Check sheet for the drawn part. Datum: minimum x, y, z corner. Units: mm. A direction names the side the tool comes from. Give positions to 0.01 mm unless a question says otherwise; leave off trailing zeros. Order: outer loops, then holes, each group sorted by start corner. A loop starts at its lowest first (then second) coordinate and runs counter-clockwise, first axis right, second up.
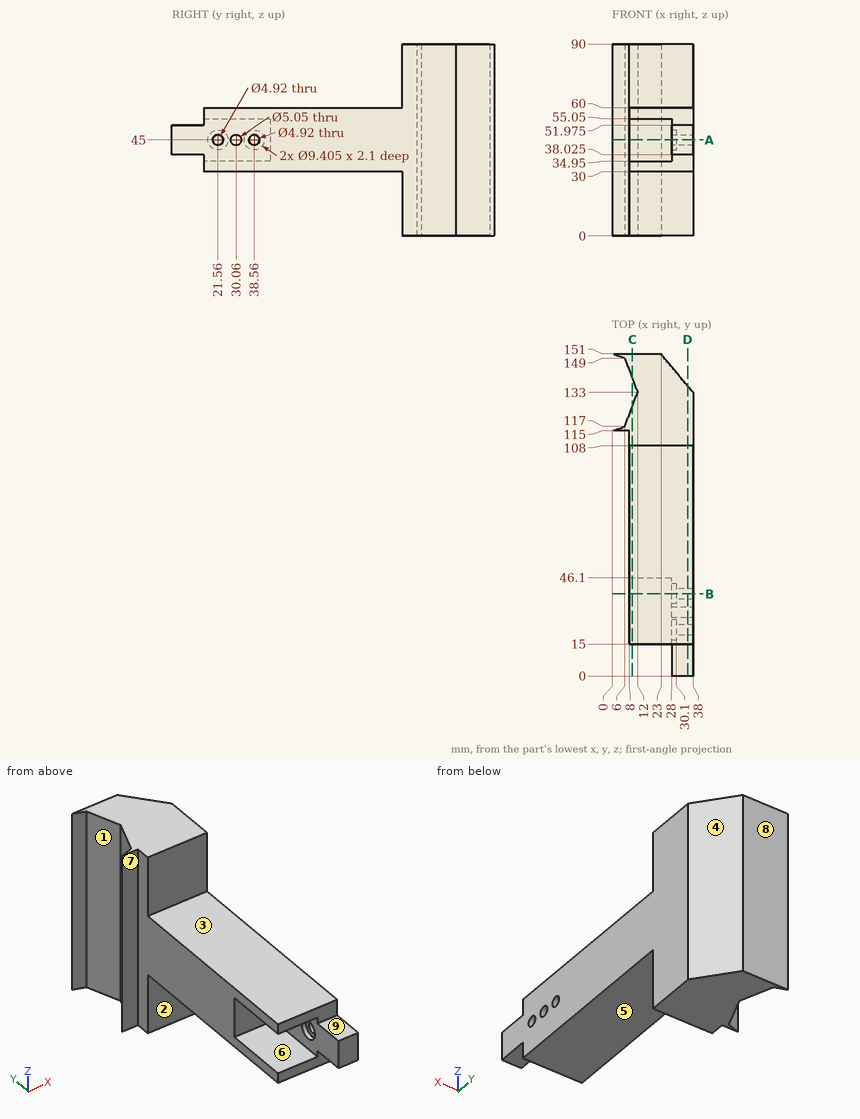
(1) Section check C-C, the plane x = 9.5. Enter the section's corners in (y, z).
Solved:
outline: (15, 30) - (108, 30) - (108, 0) - (126.33, 0) - (126.33, 90) - (108, 90) - (108, 60) - (15, 60) - (15, 55.05) - (46.1, 55.05) - (46.1, 34.95) - (15, 34.95) - close; (139.67, 0) - (151, 0) - (151, 90) - (139.67, 90) - close
(2) Section check D-D, the plane x = 35.5. Enter the section's corners in (y, z) (3 decimals).
Solved:
outline: (0, 38.025) - (15, 38.025) - (15, 30) - (108, 30) - (108, 0) - (136, 0) - (136, 90) - (108, 90) - (108, 60) - (15, 60) - (15, 51.975) - (0, 51.975) - close; hole circle Ø4.92 at (21.56, 45); hole circle Ø5.05 at (30.06, 45); hole circle Ø4.92 at (38.56, 45)
(3) Release check for a two-part mould opening along Y. For the marked faces 1, 2, 3 and 4 record: pulls with the +Y half, pulls with the -Y half, needs draft (parallel to the pull), parting line crosses it, or undercut.
Solved:
face 1: undercut
face 2: pulls with the -Y half
face 3: needs draft
face 4: pulls with the +Y half
(4) Scan lines: line 1 (Y direction, x = 33.5, z = 45) (3 decimals); line 2 (Z direction, x = 29, y = 21); line 3 (Z direction, x = 32, y = 21.56). Record each from-to range of solid material in increasing order.
Solved:
line 1: y = 0 to 19.1, 24.02 to 27.535, 32.585 to 36.1, 41.02 to 138.4
line 2: z = 30 to 40.33, 49.67 to 60
line 3: z = 30 to 42.54, 47.46 to 60
(5) Section check B-B, the plane y = 38.56. Enter the section's corners in (x, z), then the cut area to 3 significant figures.
Solved:
outline: (8, 30) - (38, 30) - (38, 42.54) - (30.1, 42.54) - (30.1, 40.3) - (28, 40.3) - (28, 34.95) - (8, 34.95) - close; (8, 55.05) - (28, 55.05) - (28, 49.7) - (30.1, 49.7) - (30.1, 47.46) - (38, 47.46) - (38, 60) - (8, 60) - close
area: 439 mm2
(6) Set-up check for the marked faces 5, 6, 7, 8 and 9: record each of +Z, -Z, +X, -X, +Y, -Y from which the full face is reachable in a straight line by a thin tool's end or side.
Solved:
face 5: -Z, +X, -X, -Y
face 6: -X, -Y
face 7: +Z, -Z, -X, -Y
face 8: +Z, -Z, +X, -X, +Y
face 9: +Z, +X, -X, -Y
(7) Section check A-A, the plane z = 45. Give the number of separate pieces and of enclosed holes in the cut face, then the cut area to 3 significant figures.
Solved:
separate pieces: 4
enclosed holes: 0
area: 3,290 mm2
(8) Go/stop test with flat-tipped pins: pin 1 (2 mm diameter, centred on x = 14.5, z = 34, fed in from -Y); pin 2 (4.5 mm diameter, centred on y = 37.5, z = 43, fed in from -X); pin 3 (2 mm diameter, centred on x = 9.5, z = 44.5, fed in from -Y); pin 4 (4.5 mm diameter, centred on y = 38.56, z = 45, fed in from +X) (1 decimal). Record where each tip stops, or that it passes through.
Solved:
pin 1: stops at y = 15
pin 2: stops at x = 30.1
pin 3: stops at y = 46.1
pin 4: passes through
